Input: part model. Units: mm. Frame: model coordinates. Face numbers are marked on the shaded views. Round coordinates to 2 decimals unless told otherwise and drop trailing zeros. Loops run counter-clockwise (first coordinate to the right, second up) from the corner with the lowest first, then second, coordinate; pieces in that order, holes last.
(1) Cut plane C-C, the plane z = 34. Output: boundary loops of the cut face in (x, y), and give its area (3 significant figures).
(2) Line query: line 1 (Y direction, x = 29, z = 32.5); line 2 (Z direction, x = 30, y = 5.5); line 3 (X direction, y = 13, z = 0). Output: solid intervals per line, ascending.
(3) Cut plane A-A, the plane z = -60. Output: boundary loops of the cut face in (x, y) (3 decimals), and give its area (3 significant figures).
(4) Cut plane D-D, the plane z = 63. Output: boundary loops of the cut face in (x, y).
(5) First-contact query: pin 1 Ø1 at (x, y) = (41.5, 19) entering from +Z; pin 2 Ø12 at (y, z) = (5, 16.5) entering from -X; pin 3 Ø1 at (y, z) = (22, -6.5) entering from +X. Flat tips, straight axial feed; report the tip coordinate or a pass-through.
(6) Cut plane B-B, the plane x = 63.5. Output: boundary loops of the cut face in (y, z).
(7) Draft query along Z for the marked faces 1 and 2. Return one class per face: released by +Z, released by -Z, zero draft, split by the parting line, or undercut.
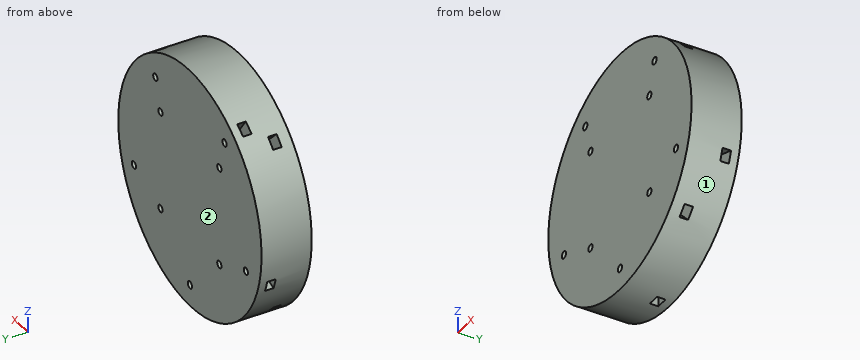
from build123d import *

# Parameters (mm, degrees)
SKETCH1_R           = 73
SKETCH1_R_2         = 2.15
BOSS_EXTRUDE1_DEPTH = 30
CUT_EXTRUDE1_START  = -5.1
CUT_EXTRUDE1_DEPTH  = 5.1
CUT_EXTRUDE2_DEPTH  = 5.1


with BuildPart() as part:
    # Sketch1 → Boss-Extrude1 (new body)
    with BuildSketch(Plane(origin=(0, 0, 0), x_dir=(1, 0, 0), z_dir=(0, 1, 0))):
        with Locations(Location((0, 0, 0), (0, 0, 270))):
            Circle(SKETCH1_R)
        with Locations(Location((30, 30, 0), (0, 0, 270))):
            Circle(SKETCH1_R_2, mode=Mode.SUBTRACT)
        with Locations(Location((-30, 30, 0), (0, 0, 90))):
            Circle(SKETCH1_R_2, mode=Mode.SUBTRACT)
        with Locations(Location((30, -30, 0), (0, 0, 90))):
            Circle(SKETCH1_R_2, mode=Mode.SUBTRACT)
        with Locations(Location((-30, -30, 0), (0, 0, 270))):
            Circle(SKETCH1_R_2, mode=Mode.SUBTRACT)
        with Locations(Location((0, 60, 0), (0, 0, 270))):
            Circle(SKETCH1_R_2, mode=Mode.SUBTRACT)
        with Locations(Location((57.063390978, 18.541019662, 0), (0, 0, 270))):
            Circle(SKETCH1_R_2, mode=Mode.SUBTRACT)
        with Locations(Location((35.267115138, -48.541019662, 0), (0, 0, 270))):
            Circle(SKETCH1_R_2, mode=Mode.SUBTRACT)
        with Locations(Location((-35.267115138, -48.541019662, 0), (0, 0, 270))):
            Circle(SKETCH1_R_2, mode=Mode.SUBTRACT)
        with Locations(Location((-57.063390978, 18.541019662, 0), (0, 0, 270))):
            Circle(SKETCH1_R_2, mode=Mode.SUBTRACT)
    extrude(amount=BOSS_EXTRUDE1_DEPTH)

    # Sketch2 → Cut-Extrude1 (cut)
    with BuildSketch(Plane(origin=(0, 12, 0), x_dir=(1, 0, 0), z_dir=(0, 1, 0)).offset(CUT_EXTRUDE1_START)):
        with BuildLine():
            Line((-27.040199894, 27.040199894), (-25.956837865, 31.083362029))
            Line((-25.956837865, 31.083362029), (-28.916637971, 34.043162135))
            Line((-28.916637971, 34.043162135), (-48.991851025, 54.118375189))
            ThreePointArc((-48.991851025, 54.118375189), (-51.618795027, 51.618795027), (-54.118375189, 48.991851025))
            Line((-54.118375189, 48.991851025), (-34.043162135, 28.916637971))
            Line((-34.043162135, 28.916637971), (-31.083362029, 25.956837865))
            Line((-31.083362029, 25.956837865), (-27.040199894, 27.040199894))
        make_face()
        with BuildLine():
            Line((28.916637971, 34.043162135), (25.956837865, 31.083362029))
            Line((25.956837865, 31.083362029), (27.040199894, 27.040199894))
            Line((27.040199894, 27.040199894), (31.083362029, 25.956837865))
            Line((31.083362029, 25.956837865), (34.043162135, 28.916637971))
            Line((34.043162135, 28.916637971), (54.118375189, 48.991851025))
            ThreePointArc((54.118375189, 48.991851025), (51.618795027, 51.618795027), (48.991851025, 54.118375189))
            Line((48.991851025, 54.118375189), (28.916637971, 34.043162135))
        make_face()
        with BuildLine():
            Line((34.043162135, -28.916637971), (31.083362029, -25.956837865))
            Line((31.083362029, -25.956837865), (27.040199894, -27.040199894))
            Line((27.040199894, -27.040199894), (25.956837865, -31.083362029))
            Line((25.956837865, -31.083362029), (28.916637971, -34.043162135))
            Line((28.916637971, -34.043162135), (48.991851025, -54.118375189))
            ThreePointArc((48.991851025, -54.118375189), (51.618795027, -51.618795027), (54.118375189, -48.991851025))
            Line((54.118375189, -48.991851025), (34.043162135, -28.916637971))
        make_face()
        with BuildLine():
            Line((-28.916637971, -34.043162135), (-25.956837865, -31.083362029))
            Line((-25.956837865, -31.083362029), (-27.040199894, -27.040199894))
            Line((-27.040199894, -27.040199894), (-31.083362029, -25.956837865))
            Line((-31.083362029, -25.956837865), (-34.043162135, -28.916637971))
            Line((-34.043162135, -28.916637971), (-54.118375189, -48.991851025))
            ThreePointArc((-54.118375189, -48.991851025), (-51.618795027, -51.618795027), (-48.991851025, -54.118375189))
            Line((-48.991851025, -54.118375189), (-28.916637971, -34.043162135))
        make_face()
    extrude(amount=CUT_EXTRUDE1_DEPTH, mode=Mode.SUBTRACT)

    # Sketch4 → Cut-Extrude2 (cut)
    with BuildSketch(Plane(origin=(0, 20, 0), x_dir=(1, 0, 0), z_dir=(0, 1, 0))):
        with BuildLine():
            Line((-3.625, 62.092894726), (-3.625, 72.909940166))
            ThreePointArc((-3.625, 72.909940166), (0, 73), (3.625, 72.909940166))
            Line((3.625, 72.909940166), (3.625, 62.092894726))
            Line((3.625, 62.092894726), (3.625, 57.907105274))
            Line((3.625, 57.907105274), (0, 55.814210548))
            Line((0, 55.814210548), (-3.625, 57.907105274))
            Line((-3.625, 57.907105274), (-3.625, 62.092894726))
        make_face()
        with BuildLine():
            Line((56.193116415, 14.446699753), (60.174038749, 15.740179829))
            Line((60.174038749, 15.740179829), (70.461660302, 19.082830699))
            ThreePointArc((70.461660302, 19.082830699), (69.42712569, 22.558240589), (68.221287093, 25.977990442))
            Line((68.221287093, 25.977990442), (57.93366554, 22.635339572))
            Line((57.93366554, 22.635339572), (53.952743206, 21.341859496))
            Line((53.952743206, 21.341859496), (53.082468644, 17.247539587))
            Line((53.082468644, 17.247539587), (56.193116415, 14.446699753))
        make_face()
        with BuildLine():
            Line((31.104255879, -48.978553801), (33.564601187, -52.364928603))
            Line((33.564601187, -52.364928603), (39.92270097, -61.116102193))
            ThreePointArc((39.92270097, -61.116102193), (42.908323417, -59.058240589), (45.78807418, -56.854659114))
            Line((45.78807418, -56.854659114), (39.429974397, -48.103485524))
            Line((39.429974397, -48.103485524), (36.969629088, -44.717110722))
            Line((36.969629088, -44.717110722), (32.806769829, -45.154644861))
            Line((32.806769829, -45.154644861), (31.104255879, -48.978553801))
        make_face()
        with BuildLine():
            Line((-36.969629088, -44.717110722), (-39.429974397, -48.103485524))
            Line((-39.429974397, -48.103485524), (-45.78807418, -56.854659114))
            ThreePointArc((-45.78807418, -56.854659114), (-42.908323417, -59.058240589), (-39.92270097, -61.116102193))
            Line((-39.92270097, -61.116102193), (-33.564601187, -52.364928603))
            Line((-33.564601187, -52.364928603), (-31.104255879, -48.978553801))
            Line((-31.104255879, -48.978553801), (-32.806769829, -45.154644861))
            Line((-32.806769829, -45.154644861), (-36.969629088, -44.717110722))
        make_face()
        with BuildLine():
            Line((-53.952743206, 21.341859496), (-57.93366554, 22.635339572))
            Line((-57.93366554, 22.635339572), (-68.221287093, 25.977990442))
            ThreePointArc((-68.221287093, 25.977990442), (-69.42712569, 22.558240589), (-70.461660302, 19.082830699))
            Line((-70.461660302, 19.082830699), (-60.174038749, 15.740179829))
            Line((-60.174038749, 15.740179829), (-56.193116415, 14.446699753))
            Line((-56.193116415, 14.446699753), (-53.082468644, 17.247539587))
            Line((-53.082468644, 17.247539587), (-53.952743206, 21.341859496))
        make_face()
    extrude(amount=CUT_EXTRUDE2_DEPTH, mode=Mode.SUBTRACT)


solid = part.part
Reported:
1. outline: (-64.6, 0) - (64.6, 0) - (64.6, 30) - (-64.6, 30) - close; hole (-39.13, 6.9) - (-28.87, 6.9) - (-28.87, 12) - (-39.13, 12) - close; hole (28.87, 6.9) - (39.13, 6.9) - (39.13, 12) - (28.87, 12) - close
1. area: 3,770 mm2
2. line 1: y = 0 to 6.9, 12 to 30
2. line 2: z = -66.55 to -32.15, -27.85 to 27.85, 32.15 to 66.55
2. line 3: x = -73 to 73
3. outline: (-41.581, 0) - (-2.15, 0) - (-2.15, 20) - (-3.625, 20) - (-3.625, 25.1) - (-2.15, 25.1) - (-2.15, 30) - (-41.581, 30) - close; (2.15, 0) - (41.581, 0) - (41.581, 30) - (2.15, 30) - (2.15, 25.1) - (3.625, 25.1) - (3.625, 20) - (2.15, 20) - close
3. area: 2,350 mm2
4. outline: (-36.88, 0) - (36.88, 0) - (36.88, 30) - (-36.88, 30) - close
5. pin 1: stops at z = 60.4
5. pin 2: stops at x = -72.24
5. pin 3: stops at x = 72.75
6. outline: (0, -36.01) - (30, -36.01) - (30, 36.01) - (0, 36.01) - close; hole (20, -24.44) - (25.1, -24.44) - (25.1, -16.82) - (20, -16.82) - close
7. face 1: split by the parting line
7. face 2: zero draft
